Could you check a few things on this drawing? It's one solid part, dimensions in mm from its lowest x, y, z. A direction names the side the tool comes from. Coordinates: 2 decimals unless noted, no trailing zeros. Write each loop counter-clockwise with the first axis right and the second up, starting at its lowest first coordinate (ties: lowest second). Pieces come first, ordered by that corner, then holes. Notation, with made-up numbers: M -30.75,61 L 6.25,61 A26 ccw 6.25,95 Z; hole C -20.5,10.25 d1. An arc over 180 degrees is marked long. Use a Markdown table: item, result.
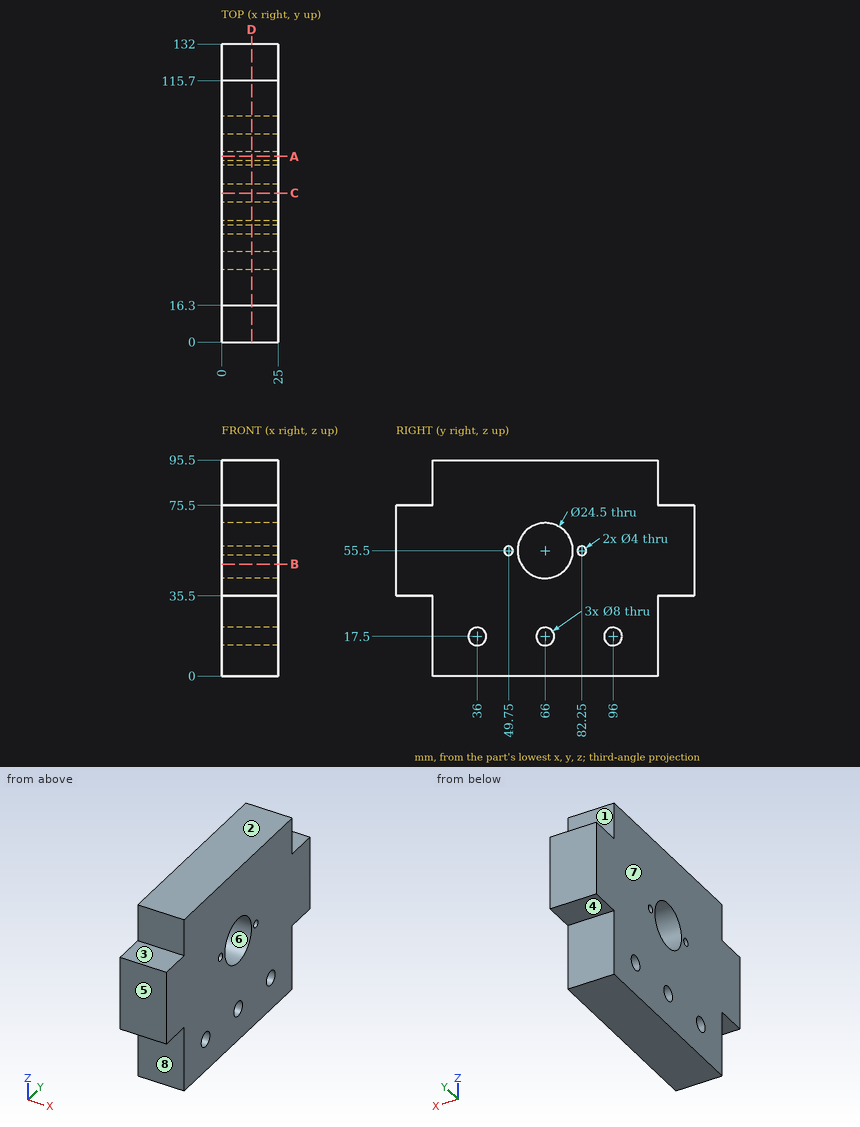
1. Suppose I cut it at B-B on z = 49.5. Write out the boundary of the cut face in (x, y), and give its area (3 significant figures).
Answers follow:
| item | result |
|---|---|
| outline | M 0,0 L 25,0 L 25,55.32 L 0,55.32 Z; M 0,76.68 L 25,76.68 L 25,132 L 0,132 Z |
| area | 2,770 mm2 |
2. Suppose I cut it at C-C on y = 66. Write out the boundary of the cut face in (x, z), and give its area (4 significant figures).
Answers follow:
| item | result |
|---|---|
| outline | M 0,0 L 25,0 L 25,13.5 L 0,13.5 Z; M 0,21.5 L 25,21.5 L 25,43.25 L 0,43.25 Z; M 0,67.75 L 25,67.75 L 25,95.5 L 0,95.5 Z |
| area | 1,575 mm2 |
3. Which directions (+Z, -Z, +X, -X, +Y, -Y) give clear straight access to the entire face, cutting with the end or side of a thin tool? Please do the marked faces 1, 2, 3, 4 and 5.
Answers follow:
| item | result |
|---|---|
| face 1 | +Z, +X, -X, +Y |
| face 2 | +Z, +X, -X, +Y, -Y |
| face 3 | +Z, +X, -X, -Y |
| face 4 | -Z, +X, -X, +Y |
| face 5 | +Z, -Z, +X, -X, -Y |
4. Will these pins go through, and if not, where does the flat tip stop? pin 1 Ø10 at (x, z) = (12, 81) entering from -Y; pin 2 Ø10 at (x, z) = (8, 81.5) entering from +Y; pin 3 Ø5 at (x, y) = (12, 11.5) entering from +Z; pin 4 Ø7 at (y, z) = (66, 17.5) entering from -X.
Answers follow:
| item | result |
|---|---|
| pin 1 | stops at y = 16.3 |
| pin 2 | stops at y = 115.7 |
| pin 3 | stops at z = 75.5 |
| pin 4 | passes through |
5. We'd pull the mould along Y, two halves only. Please class the marked faces 6, 7 and 8: +Y half, -Y half, draft (parallel to the pull), parting line (faces both ways), or undercut.
Answers follow:
| item | result |
|---|---|
| face 6 | undercut |
| face 7 | draft |
| face 8 | -Y half |
6. Suppose I cut it at A-A on y = 82.25. Write out the boundary of the cut face in (x, z).
Answers follow:
| item | result |
|---|---|
| outline | M 0,0 L 25,0 L 25,53.5 L 0,53.5 Z; M 0,57.5 L 25,57.5 L 25,95.5 L 0,95.5 Z |
7. Suppose I cut it at D-D on x = 13.25. Write out the boundary of the cut face in (y, z), and give its area (3 significant figures).
Answers follow:
| item | result |
|---|---|
| outline | M 0,35.5 L 16.3,35.5 L 16.3,0 L 115.7,0 L 115.7,35.5 L 132,35.5 L 132,75.5 L 115.7,75.5 L 115.7,95.5 L 16.3,95.5 L 16.3,75.5 L 0,75.5 Z; hole C 36,17.5 d8; hole C 49.75,55.5 d4; hole C 66,55.5 d24.5; hole C 66,17.5 d8; hole C 82.25,55.5 d4; hole C 96,17.5 d8 |
| area | 10,100 mm2 |
8. I need wall thicknesses on probe 1 along Z at (x, y) = (12, 66); probe 2 along Y at (x, z) = (9.75, 18); probe 3 along Z at (x, y) = (20, 96). Which ranges of each line are inside material? Lowest first, please.
Answers follow:
| item | result |
|---|---|
| probe 1 | z = 0 to 13.5, 21.5 to 43.25, 67.75 to 95.5 |
| probe 2 | y = 16.3 to 32.03, 39.97 to 62.03, 69.97 to 92.03, 99.97 to 115.7 |
| probe 3 | z = 0 to 13.5, 21.5 to 95.5 |
